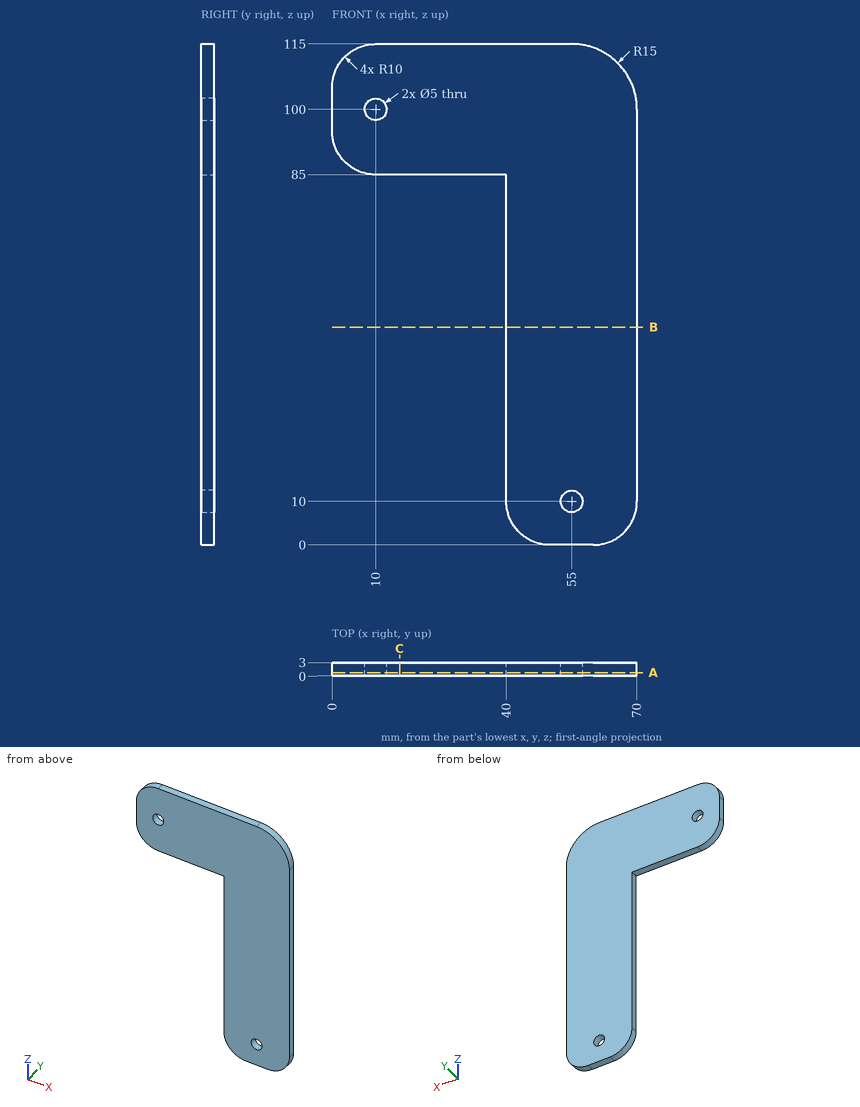
Geometry: see drawing. Coordinates: mm, zero at the bounding-box minimum. Coordinates: 2 decimals unless noted, no trailing zeros. Write each loop counter-clockwise with the first axis right and the second up, starting at its lowest first coordinate (ties: lowest second). Pieces come first, ordered by that corner, then holes. Notation, with made-up numbers: M -18.5,51.25 L 32.5,51.25 A30 ccw 32.5,88.25 Z; hole C -21,11.5 d1. An arc over 180 degrees is marked long. Use CSV: the item, a comma, the result in double quotes. Start each with the question number.
1. Ray query, probe 1 along X at (y, z) = (0.6, 100); probe 2 along X at (y, z) = (1.05, 10); probe 3 along X at (y, z) = (0.6, 65). Return the intervals inside material, ascending.
2. Cut plane B-B on z = 50. Return the cut outline in (x, y).
3. Cut plane C-C on x = 15.5. Return the cut outline in (y, z).
4. Cut plane A-A on y = 0.75. Return the cut outline in (x, z), plus the area to 3 significant figures.
Entries:
1,probe 1,"0 to 7.5, 12.5 to 70"
1,probe 2,"40 to 52.5, 57.5 to 70"
1,probe 3,"40 to 70"
2,outline,"M 40,0 L 70,0 L 70,3 L 40,3 Z"
3,outline,"M 0,85 L 3,85 L 3,115 L 0,115 Z"
4,outline,"M 0,95 A10 ccw 10,85 L 40,85 L 40,10 A10 ccw 50,0 L 60,0 A10 ccw 70,10 L 70,100 A15 ccw 55,115 L 10,115 A10 ccw 0,105 Z; hole C 10,100 d5; hole C 55,10 d5"
4,area,"4,480 mm²"
